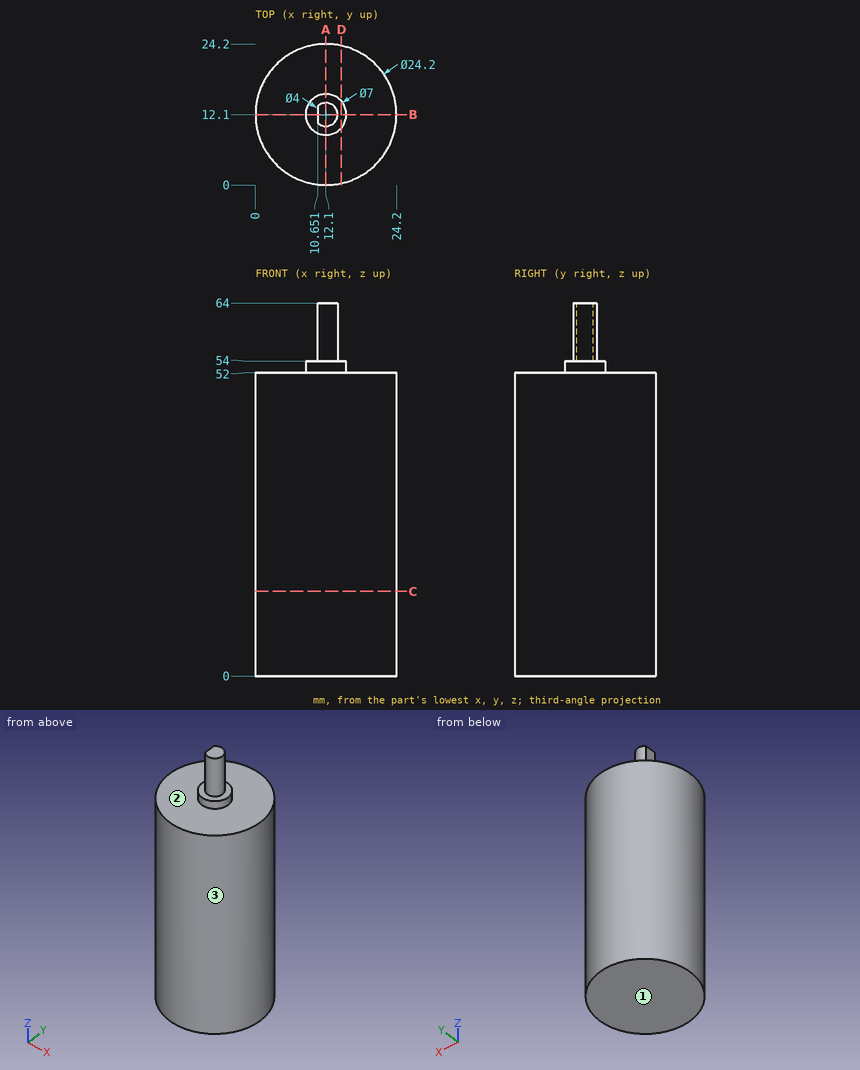
Part print with two shaded views. Sizes in mm from the minimum x, y, z corner. Round coordinates to 2 decimals unless told otherwise and drop trailing zeros. Write each loop counter-clockwise with the first axis right and the second up, starting at its lowest first coordinate (ties: lowest second). Pieces come first, ordered by that corner, then holes. Notation, with made-up numbers: (30, 15) -> (34, 15) arc R22 cw to (34, 52) -> close; hole circle Ø5 at (19.5, -35.5). An arc over 180 degrees is marked (long way). Put each result on its own line as item: value.
Item 1: Slice it at A-A, the plane x = 12.1. Give the cut face in (y, z).
Here are the results:
outline: (0, 0) -> (24.2, 0) -> (24.2, 52) -> (15.6, 52) -> (15.6, 54) -> (14.1, 54) -> (14.1, 64) -> (10.1, 64) -> (10.1, 54) -> (8.6, 54) -> (8.6, 52) -> (0, 52) -> close
Item 2: Slice it at D-D, the plane x = 14.75. Give the cut face in (y, z), plus the area to 3 significant figures.
Here are the results:
outline: (0.29, 0) -> (23.91, 0) -> (23.91, 52) -> (14.39, 52) -> (14.39, 54) -> (9.81, 54) -> (9.81, 52) -> (0.29, 52) -> close
area: 1,240 mm^2
Item 3: Flat gauge pins, fed straight in: P1, Ø1, axis at y = 5, z = 27, coming from the +X side; P2, Ø1.5, axis at x = 7, y = 13, coming from the +Z side; P3, Ø8, axis at y = 4, z = 15, coming from the -X side. Where does each tip first touch, or does it go through?
Here are the results:
P1: stops at x = 22.24
P2: stops at z = 52
P3: stops at x = 0.72
Item 4: Two-plate mould, pull along Z, no slides. Class the marked faces 1, 2 and 3: pulls with the +Z half, pulls with the -Z half, needs draft (parallel to the pull), parting line crosses it, or undercut.
Here are the results:
face 1: pulls with the -Z half
face 2: pulls with the +Z half
face 3: needs draft
Item 5: Slice it at B-B, the plane y = 12.1. Give the cut face in (x, z).
Here are the results:
outline: (0, 0) -> (24.2, 0) -> (24.2, 52) -> (15.6, 52) -> (15.6, 54) -> (14.1, 54) -> (14.1, 64) -> (10.65, 64) -> (10.65, 54) -> (8.6, 54) -> (8.6, 52) -> (0, 52) -> close
Item 6: Slice it at C-C, the plane z = 14.5. Give the cut face in (x, y).
Here are the results:
outline: circle Ø24.2 at (12.1, 12.1)
Item 7: Wall check: probe 1 along Z at (x, y) = (10.75, 8.25); probe 2 along Y at (x, z) = (12.5, 32); probe 3 along Y at (x, z) = (20.25, 33) (1 decimal). Give the ranges that are in metal, low to high. Write a range as from..to.
Here are the results:
probe 1: z = 0..52
probe 2: y = 0.01..24.19
probe 3: y = 3.2..21
